Work out the finished part from the listing and answer in its coordinate system (mm). Face numbers are marked on the shaded views. A direction names the side the tool comes from. Round coordinates to 2 decimals unless told otherwise and drop trailing zeros. Write each loop counter-clockwise with the first axis right and the second up, starting at its lowest first coordinate (ties: lowest second). Pieces come first, ordered by that corner, then holes. Notation, with made-up numbers: (16, 32) - (61, 32) arc R14 ccw to (61, 42) - close; hole circle Ø4 at (80.25, 53.25). An arc over 180 degrees is marked (long way). Answer as a JSON object with one key per item and string values.
```python
from build123d import *

# Parameters (mm, degrees)
TUBE_PROFILE_R          = 7.35
TUBE_PROFILE_R_2        = 6.35
EXTRUDE_THIN_REACH      = 31.111
EXTRUDE_THIN_END_RADIUS = 7.35
EXTRUDE_THIN_START      = -12.7
PROFILE_R               = 7.35
PROFILE_R_2             = 6.35
CUT_EXTRUDE_START       = -7.35
PROFILE_2_R             = 6.35
CUT_EXTRUDE_DEPTH       = 7.35


with BuildPart() as part:
    # Tube: sweep along a path in Path
    with BuildLine(Plane(origin=(0, 0, 0), x_dir=(0, 0, -1), z_dir=(1, 0, 0))) as tube_path:
        Line((-12.7, 0), (12.7, 0))
    # Tube profile (on start of the path) → Tube (sweep)
    with BuildSketch(Plane(origin=(0, 0, 12.7), x_dir=(0, -1, 0), z_dir=(0, 0, -1))):
        Circle(TUBE_PROFILE_R)
        Circle(TUBE_PROFILE_R_2, mode=Mode.SUBTRACT)
    sweep(path=tube_path.line)

    # Extrude-Thin: up to this cylinder (the profile starts outside it)
    extrude_thin_end = Plane(origin=(0, 0, 0), z_dir=(0, 0, -1)) * Cylinder(EXTRUDE_THIN_END_RADIUS, 77.922, mode=Mode.PRIVATE)
    # Profile → Extrude-Thin (add, up to the surface)
    with BuildSketch(Plane(origin=(0, 0, 0), x_dir=(1, 0, 0), z_dir=(0, 1, 0)).offset(EXTRUDE_THIN_START), mode=Mode.PRIVATE) as extrude_thin_sk1:
        Circle(PROFILE_R)
        Circle(PROFILE_R_2, mode=Mode.SUBTRACT)
    extrude_thin_tool1 = extrude(extrude_thin_sk1.sketch, amount=EXTRUDE_THIN_REACH, mode=Mode.PRIVATE) - extrude_thin_end
    add(extrude_thin_tool1.solids().sort_by_distance((-7.142111, -12.7, 0))[0])

    # Profile<2> → Cut-Extrude (cut)
    with BuildSketch(Plane(origin=(0, 0, 0), x_dir=(1, 0, 0), z_dir=(0, 1, 0)).offset(CUT_EXTRUDE_START)):
        with Locations(Location((0, 0, 0), (0, 0, 180))):
            Circle(PROFILE_2_R)
    extrude(amount=CUT_EXTRUDE_DEPTH, mode=Mode.SUBTRACT)


solid = part.part
```
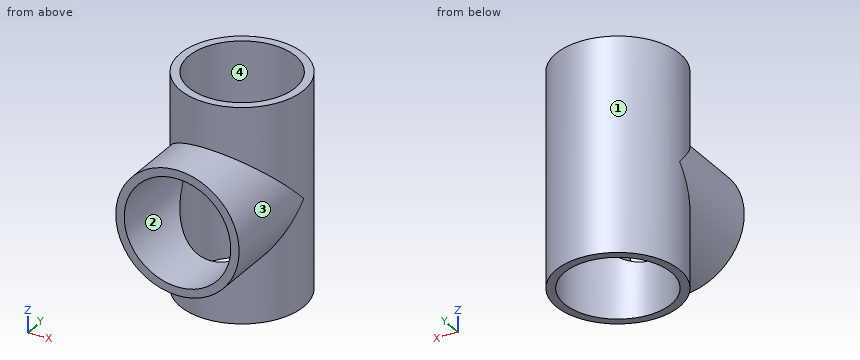
Item 1: A cutting plane is placed at C-C (y = -6.75). Write down the section's boundary in (x, z).
Results found:
{"outline": "(-2.91, -12.7) - (2.91, -12.7) - (2.91, -6.75) arc R7.35 ccw to (2.91, 6.75) - (2.91, 12.7) - (-2.91, 12.7) - (-2.91, 6.75) arc R7.35 ccw to (-2.91, -6.75) - close; hole circle Ø12.7 at (0, 0)"}
Item 2: For the marked faces 3 and 4, determine the directions among +Z, -Z, +X, -X, +Y, -Y from which every point of the face is accessible in a straight line to the end or side of a thin tool.
Results found:
{"face 3": "-Y", "face 4": "+Z, -Z"}
Item 3: Determine the mould class of the marked faces 1 and 2 for opening direction X: pulls with the +X half, pulls with the -X half, needs draft (parallel to the pull), parting line crosses it, or undercut.
Results found:
{"face 1": "parting line crosses it", "face 2": "undercut"}
Item 4: Consider line 1 along X through (y, z) = (0, 2). Determine where the line is inside the solid, lowest interval first.
Results found:
{"line 1": "-7.35 to -6.35, 6.35 to 7.35"}
Item 5: Each of these flat-tipped pins is pushed along its axis until it touches: P1, Ø1, axis at y = 4, z = -5.5, coming from the +X side; P2, Ø1, axis at x = -5.5, y = -10, coming from the +Z side; P3, Ø2, axis at y = -4, z = -5.5, coming from the -X side. Where does it stop, or does it pass through?
Results found:
{"P1": "x = 6.46", "P2": "z = 5.39", "P3": "x = -6.71"}
Item 6: A cutting plane is placed at B-B (y = -2.25). Write down the section's boundary in (x, z), and give its area (3 significant figures).
Results found:
{"outline": "(-7, -12.7) - (-5.94, -12.7) - (-5.94, -2.25) arc R6.35 cw to (-5.94, 2.25) - (-5.94, 12.7) - (-7, 12.7) - (-7, 2.25) arc R7.35 ccw to (-7, -2.25) - close; (5.94, -12.7) - (7, -12.7) - (7, -2.25) arc R7.35 ccw to (7, 2.25) - (7, 12.7) - (5.94, 12.7) - (5.94, 2.25) arc R6.35 cw to (5.94, -2.25) - close", "area": "53.4 mm²"}
Item 7: A cutting plane is placed at D-D (z = 6.75). Write down the section's boundary in (x, y).
Results found:
{"outline": "(-2.91, -12.7) - (2.91, -12.7) - (2.91, -6.75) arc R7.35 ccw (long way) to (-2.91, -6.75) - close; hole circle Ø12.7 at (0, 0)"}
